Check sheet for the modelled part. Datum: model origin and axes. Units: mm. Face numbers are marked on the shaded views. Round coordinates to 2 decimals unless told otherwise and drop trailing zeros. Loops run counter-clockwise (first coordinate to the right, second up) from the corner with the lowest first, then second, coordinate; pieces in that order, holes last. Notation, with made-up numbers: (61.5, 34) - (68.5, 34) arc R19 ccw to (68.5, 50) - close; hole circle Ø5 at (76.25, -15.75). An arc over 180 degrees is marked (long way). Answer in a Markdown table with one row per item. Add a question column.
(1) Cross-section at B-B on z = 9.5. Enter the section's corners in (x, y), then the cut area to 3 significant figures.
(2) Mould release check, pull along Y, two halves, no side actions. Record for the marked faces 1, 2 and 3: +Y half, -Y half, draft (parallel to the pull), parting line (faces both ways), or undercut.
(3) Cross-section at A-A on y = 100. Enter the section's corners in (x, z).
(4) Cross-section at D-D on x = 238. Enter the section's corners in (y, z), then the cut area to 3 significant figures.
(5) Gauge pin test, flat ends, axial feed: pin 1 (5 mm diameter, centred on x = 228.5, y = 95.5, fed in from -Z); pin 2 (6 mm diameter, centred on x = 229.88, y = 100, fed in from +Z); pin 3 (1.5 mm diameter, centred on y = 106.5, z = 15, fed in from +X); pin 4 (5 mm diameter, centred on x = 230.5, z = 16.5, fed in from -Y). Record the tip position at first contact, or that the pin passes through.
(6) Thickness scan on line 1 along Z through (x, y) = (226.25, 100); line 2 along Y through (x, z) = (227.75, 16.5); line 3 along Y through (x, z) = (229.25, 3.25). Record the ranges inside material, lowest first.
(7) Cross-section at C-C on z = 18.25. Enter the section's corners in (x, y), then the cut area to 3 significant figures.
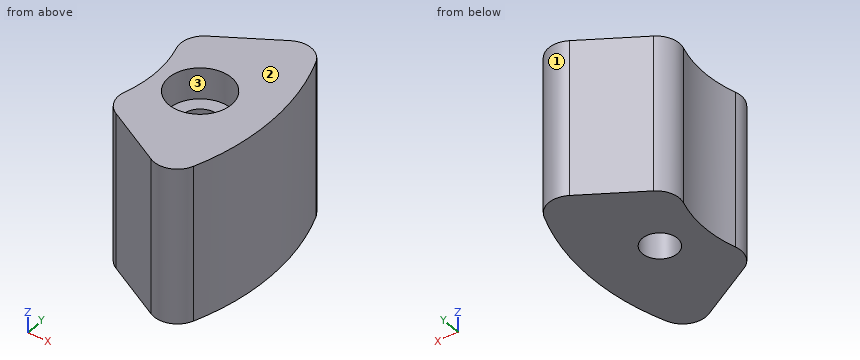
from build123d import *

# Parameters (mm, degrees)
RESSALTO_EXTRUS_O1_DEPTH          = 20
REBAIXO_PARA_SHCS_M41_D           = 4.5
REBAIXO_PARA_SHCS_M41_CBORE_D     = 8
REBAIXO_PARA_SHCS_M41_CBORE_DEPTH = 4


with BuildPart() as part:
    # Esboço1 → Ressalto-extrusão1 (new body)
    with BuildSketch(Plane.XY):
        with BuildLine():
            Line((224.973932781, 108.136324985), (232.491448563, 112.476564746))
            ThreePointArc((232.491448563, 112.476564746), (234.984464913, 112.709375061), (236.785753669, 110.970211474))
            ThreePointArc((236.785753669, 110.970211474), (238.85268513, 100), (236.785753669, 89.029788526))
            ThreePointArc((236.785753669, 89.029788526), (234.984464913, 87.290624939), (232.491448563, 87.523435254))
            Line((232.491448563, 87.523435254), (224.973932781, 91.863675015))
            ThreePointArc((224.973932781, 91.863675015), (223.679685252, 93.369880929), (223.609856165, 95.354536271))
            ThreePointArc((223.609856165, 95.354536271), (224.317111682, 100), (223.609856165, 104.645463729))
            ThreePointArc((223.609856165, 104.645463729), (223.679685252, 106.630119071), (224.973932781, 108.136324985))
        make_face()
    extrude(amount=RESSALTO_EXTRUS_O1_DEPTH)

    # Rebaixo para SHCS M41 (through all)
    with Locations(Plane.XY.offset(20)):
        with Locations((229.88140452, 100)):
            CounterBoreHole(REBAIXO_PARA_SHCS_M41_D / 2, REBAIXO_PARA_SHCS_M41_CBORE_D / 2, REBAIXO_PARA_SHCS_M41_CBORE_DEPTH)


solid = part.part
Answers:
| question | item | result |
|---|---|---|
| 1 | outline | (223.61, 95.35) arc R3 ccw to (224.97, 91.86) - (232.49, 87.52) arc R3 ccw to (236.79, 89.03) arc R30.15 ccw to (236.79, 110.97) arc R3 ccw to (232.49, 112.48) - (224.97, 108.14) arc R3 ccw to (223.61, 104.65) arc R15.61 cw to start; hole circle Ø4.5 at (229.88, 100) |
| 1 | area | 293 mm^2 |
| 2 | face 1 | +Y half |
| 2 | face 2 | draft |
| 2 | face 3 | undercut |
| 3 | outline | (224.32, 0) - (227.63, 0) - (227.63, 16) - (225.88, 16) - (225.88, 20) - (224.32, 20) - close; (232.13, 0) - (238.85, 0) - (238.85, 20) - (233.88, 20) - (233.88, 16) - (232.13, 16) - close |
| 4 | outline | (92.88, 0) - (107.12, 0) - (107.12, 20) - (92.88, 20) - close |
| 4 | area | 285 mm^2 |
| 5 | pin 1 | stops at z = 0 |
| 5 | pin 2 | stops at z = 16 |
| 5 | pin 3 | stops at x = 238.3 |
| 5 | pin 4 | stops at y = 87.29 |
| 6 | line 1 | z = 0 to 16 |
| 6 | line 2 | y = 90.26 to 96.62, 103.38 to 109.74 |
| 6 | line 3 | y = 89.39 to 97.84, 102.16 to 110.61 |
| 7 | outline | (223.61, 95.35) arc R3 ccw to (224.97, 91.86) - (232.49, 87.52) arc R3 ccw to (236.79, 89.03) arc R30.15 ccw to (236.79, 110.97) arc R3 ccw to (232.49, 112.48) - (224.97, 108.14) arc R3 ccw to (223.61, 104.65) arc R15.61 cw to start; hole circle Ø8 at (229.88, 100) |
| 7 | area | 259 mm^2 |
